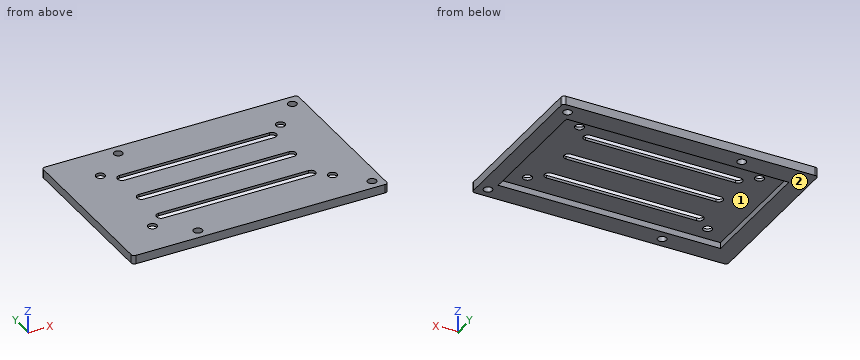
from build123d import *

# Parameters (mm, degrees)
SKETCH1_W           = 85.073492716
SKETCH1_H           = 56
SKETCH1_R           = 1.45
SKETCH1_R_2         = 1.444439883
BOSS_EXTRUDE2_DEPTH = 2.9
FILLET1_R           = 1
SKETCH2_W           = 74.073492716
SKETCH2_H           = 42
CUT_EXTRUDE1_DEPTH  = 2
SKETCH3_R           = 1.5
CUT_EXTRUDE2_DEPTH  = 13


with BuildPart() as part:
    # Sketch1 → Boss-Extrude2 (new body)
    with BuildSketch(Plane.XY):
        with Locations((0.5, -16.452272815)):
            Rectangle(SKETCH1_W, SKETCH1_H)
        with Locations((39.536746358, 8.047727185)):
            Circle(SKETCH1_R, mode=Mode.SUBTRACT)
        with Locations((39.536746358, -40.952272815)):
            Circle(SKETCH1_R, mode=Mode.SUBTRACT)
        with Locations((-18.463253642, 8.047727185)):
            Circle(SKETCH1_R, mode=Mode.SUBTRACT)
        with Locations((-18.463253642, -40.952272815)):
            Circle(SKETCH1_R_2, mode=Mode.SUBTRACT)
    extrude(amount=BOSS_EXTRUDE2_DEPTH)

    # Fillet1
    fillet1_edges = [part.edges().sort_by_distance(p)[0] for p in [
        (-42.036746358, 11.547727185, 1.45),
        (43.036746358, 11.547727185, 1.45),
        (43.036746358, -44.452272815, 1.45),
        (-42.036746358, -44.452272815, 1.45),
    ]]
    fillet(fillet1_edges, radius=FILLET1_R)

    # Sketch2 → Cut-Extrude1 (cut)
    with BuildSketch(Plane(origin=(0, 0, 0), x_dir=(-1, 0, 0), z_dir=(0, 0, -1))):
        with Locations((-1, -16.452272815)):
            Rectangle(SKETCH2_W, SKETCH2_H)
    extrude(amount=-CUT_EXTRUDE1_DEPTH, mode=Mode.SUBTRACT)

    # Sketch3 → Cut-Extrude2 (cut)
    with BuildSketch(Plane(origin=(0, 0, 2), x_dir=(-1, 0, 0), z_dir=(0, 0, -1))):
        with Locations((-31, -0.452272815)):
            Circle(SKETCH3_R)
        with Locations((-31, -32.452272815)):
            Circle(SKETCH3_R)
        with Locations((29, -32.452272815)):
            Circle(SKETCH3_R)
        with Locations((29, -0.452272815)):
            Circle(SKETCH3_R)
        with BuildLine():
            Line((-26, -2.952272815), (24, -2.952272815))
            ThreePointArc((24, -2.952272815), (25.5, -4.452272815), (24, -5.952272815))
            Line((24, -5.952272815), (-26, -5.952272815))
            ThreePointArc((-26, -5.952272815), (-27.5, -4.452272815), (-26, -2.952272815))
        make_face()
        with BuildLine():
            Line((-26, -29.952272815), (24, -29.952272815))
            ThreePointArc((24, -29.952272815), (25.5, -28.452272815), (24, -26.952272815))
            Line((24, -26.952272815), (-26, -26.952272815))
            ThreePointArc((-26, -26.952272815), (-27.5, -28.452272815), (-26, -29.952272815))
        make_face()
        with BuildLine():
            Line((-26, -14.952272815), (24, -14.952272815))
            ThreePointArc((24, -14.952272815), (25.5, -16.452272815), (24, -17.952272815))
            Line((24, -17.952272815), (-26, -17.952272815))
            ThreePointArc((-26, -17.952272815), (-27.5, -16.452272815), (-26, -14.952272815))
        make_face()
    extrude(amount=-CUT_EXTRUDE2_DEPTH, mode=Mode.SUBTRACT)


solid = part.part
For this review, take the finished solid that the model builds, in its own axes (mm). Face numbers are marked on the shaded views. Coordinates: 2 decimals unless noted, no trailing zeros. Loops run counter-clockwise (first coordinate to the right, second up) from the corner with the lowest first, then second, coordinate; pieces in that order, holes last. Notation, with made-up numbers: (62.5, -33) - (82.5, -33) arc R21 cw to (82.5, -5) - close; hole circle Ø11 at (-37.75, 3). An arc over 180 degrees is marked (long way). Return JSON: item names as keys, results as strings.
Item 1: Take a section at B-B (x = -29). Give the boundary of the cut face in (y, z), then the cut area to 3 significant figures.
Determined:
{"outline": "(-44.45, 0) - (-37.45, 0) - (-37.45, 2) - (-33.95, 2) - (-33.95, 2.9) - (-44.45, 2.9) - close; (-30.95, 2) - (-1.95, 2) - (-1.95, 2.9) - (-30.95, 2.9) - close; (1.05, 2) - (4.55, 2) - (4.55, 0) - (11.55, 0) - (11.55, 2.9) - (1.05, 2.9) - close", "area": "73.0 mm2"}
Item 2: For line 1 (Y direction, x = -29, z = 2.2); line 2 (Y direction, x = 10, z = 2.25); line 3 (Y direction, x = 34, z = 1.9), list the stretches that pass through material, from the lowest coordinate up.
Determined:
{"line 1": "y = -44.45 to -33.95, -30.95 to -1.95, 1.05 to 11.55", "line 2": "y = -44.45 to -29.95, -26.95 to -17.95, -14.95 to -5.95, -2.95 to 11.55", "line 3": "y = -44.45 to -37.45, 4.55 to 11.55"}
Item 3: Mouldability with a two-part tool opening along Y and no side actions: class the marked faces 1 and 2 as pulls with the +Y half, pulls with the -Y half, needs draft (parallel to the pull), parting line crosses it, or undercut.
Determined:
{"face 1": "undercut", "face 2": "needs draft"}
Item 4: Insertion check: pin 1 (3.5 mm diameter, centred on x = 31, y = -0.45, fed in from +Z); pin 2 (8 mm diameter, centred on x = 24.5, y = -13.5, fed in from -Z). Each pin has a flat end and moves straight along its axis. Give the tip position at first contact, or say it passes through.
Determined:
{"pin 1": "stops at z = 2.9", "pin 2": "stops at z = 2"}
Item 5: Take a section at C-C (y = -5). Give the boundary of the cut face in (x, z).
Determined:
{"outline": "(-42.04, 0) - (-36.04, 0) - (-36.04, 2) - (-25.4, 2) - (-25.4, 2.9) - (-42.04, 2.9) - close; (27.4, 2) - (38.04, 2) - (38.04, 0) - (43.04, 0) - (43.04, 2.9) - (27.4, 2.9) - close"}
Item 6: Take a section at A-A (x = -3). Give the boundary of the cut face in (y, z).
Determined:
{"outline": "(-44.45, 0) - (-37.45, 0) - (-37.45, 2) - (-29.95, 2) - (-29.95, 2.9) - (-44.45, 2.9) - close; (-26.95, 2) - (-17.95, 2) - (-17.95, 2.9) - (-26.95, 2.9) - close; (-14.95, 2) - (-5.95, 2) - (-5.95, 2.9) - (-14.95, 2.9) - close; (-2.95, 2) - (4.55, 2) - (4.55, 0) - (11.55, 0) - (11.55, 2.9) - (-2.95, 2.9) - close"}
Item 7: Take a section at D-D (y = -23). Give the boundary of the cut face in (x, z), then the cut area to 3 significant figures.
Determined:
{"outline": "(-42.04, 0) - (-36.04, 0) - (-36.04, 2) - (38.04, 2) - (38.04, 0) - (43.04, 0) - (43.04, 2.9) - (-42.04, 2.9) - close", "area": "98.6 mm2"}
